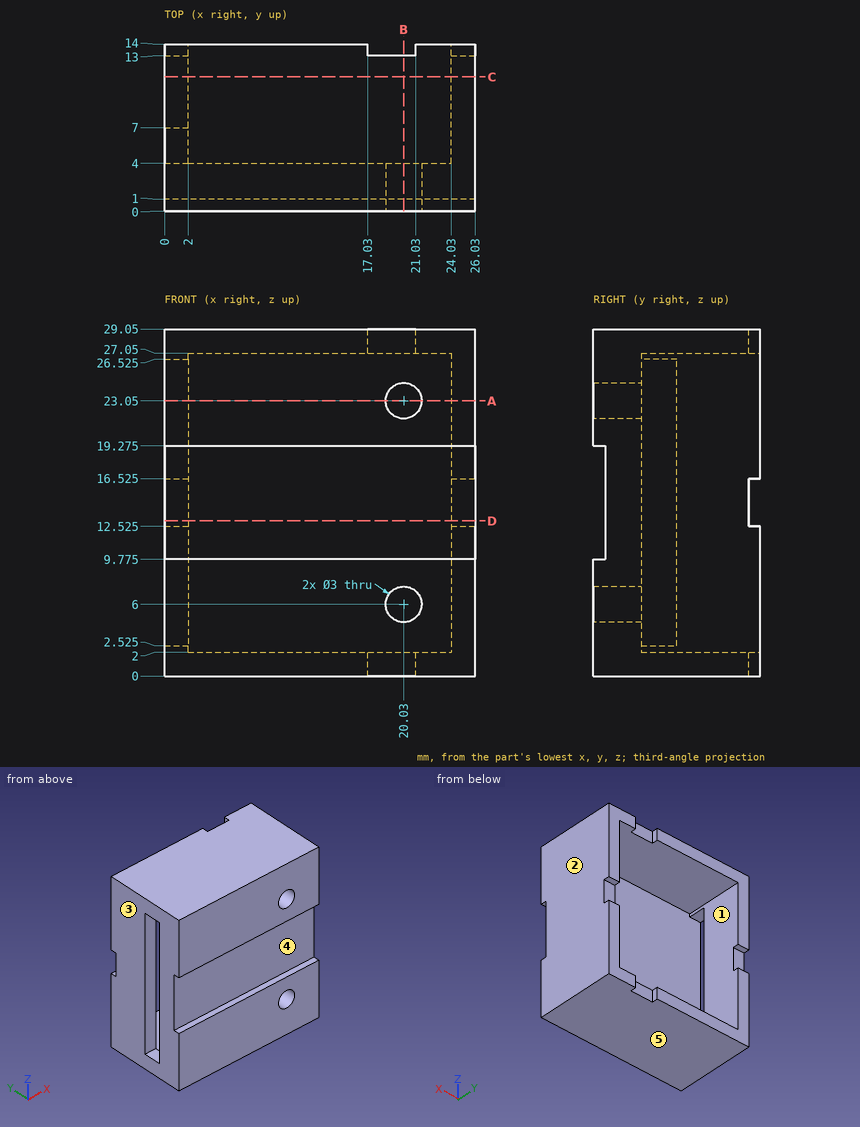
Geometry check sheet. Reference: drawing and pictorial views, mm from the part's lowest x, y, z. A direction names the side the tool comes from. Round coordinates to 2 decimals unless told otherwise and drop trailing zeros. Write each loop counter-clockwise with the first axis right and the second up, starting at its lowest first coordinate (ties: lowest second). Pieces come first, ordered by that corner, then holes.
(1) Access from +Z, -Z, +X, -X, +Y, -Y to the whole of each face (thin tool, end or side, straight path). Record for the marked faces 1 and 2.
Returned:
face 1: +Y
face 2: +Z, -Z, +X, +Y, -Y
(2) Section check B-B (x = 20.03). Enter the section's corners in (y, z) (3 decimals).
Returned:
outline: (0, 0) - (13, 0) - (13, 2) - (4, 2) - (4, 4.5) - (0, 4.5) - close; (0, 7.5) - (4, 7.5) - (4, 21.55) - (0, 21.55) - (0, 19.275) - (1, 19.275) - (1, 9.775) - (0, 9.775) - close; (0, 24.55) - (4, 24.55) - (4, 27.05) - (13, 27.05) - (13, 29.05) - (0, 29.05) - close
(3) Section check D-D (z = 13). Enter the section's corners in (x, y).
Returned:
outline: (0, 1) - (26.03, 1) - (26.03, 13) - (24.03, 13) - (24.03, 4) - (0, 4) - close; (0, 7) - (2, 7) - (2, 13) - (0, 13) - close
(4) Material ranges on line 1 (X direction, y = 1.45, z = 6); line 2 (Z direction, x = 4.5, y = 7.25); line 3 (X direction, y = 9, z = 12.75), recorded low to high.
Returned:
line 1: x = 0 to 18.53, 21.53 to 26.03
line 2: z = 0 to 2, 27.05 to 29.05
line 3: x = 0 to 2, 24.03 to 26.03
(5) Mould release check, pull along Z, two halves, no side actions. Record for the marked faces 3, 4 and 5: pulls with the +Z half, pulls with the -Z half, needs draft (parallel to the pull), parting line crosses it, or undercut.
Returned:
face 3: needs draft
face 4: undercut
face 5: pulls with the -Z half
(6) Depth check by flat-ended pin: pin 1 Ø3 at (x, z) = (20.5, 4.5) entering from -Y; pin 2 Ø5 at (x, z) = (16.5, 21.5) entering from +Y; pin 3 Ø2 at (x, z) = (18.5, 0.5) entering from +Y; pin 4 Ø2 at (x, z) = (1.5, 14.5) entering from -Y. Enter the tip coordinate at first touch or a pass-through.
Returned:
pin 1: stops at y = 0
pin 2: stops at y = 4
pin 3: stops at y = 13
pin 4: stops at y = 1
(7) Section check A-A (z = 23.05). Enter the section's corners in (x, y), plus the area to 3 significant figures.
Returned:
outline: (0, 0) - (18.53, 0) - (18.53, 4) - (0, 4) - close; (0, 7) - (2, 7) - (2, 14) - (0, 14) - close; (21.53, 0) - (26.03, 0) - (26.03, 14) - (24.03, 14) - (24.03, 4) - (21.53, 4) - close
area: 126 mm2
(8) Section check C-C (y = 11.25). Enter the section's corners in (x, z).
Returned:
outline: (0, 0) - (26.03, 0) - (26.03, 29.05) - (0, 29.05) - close; hole (2, 2) - (24.03, 2) - (24.03, 27.05) - (2, 27.05) - close
